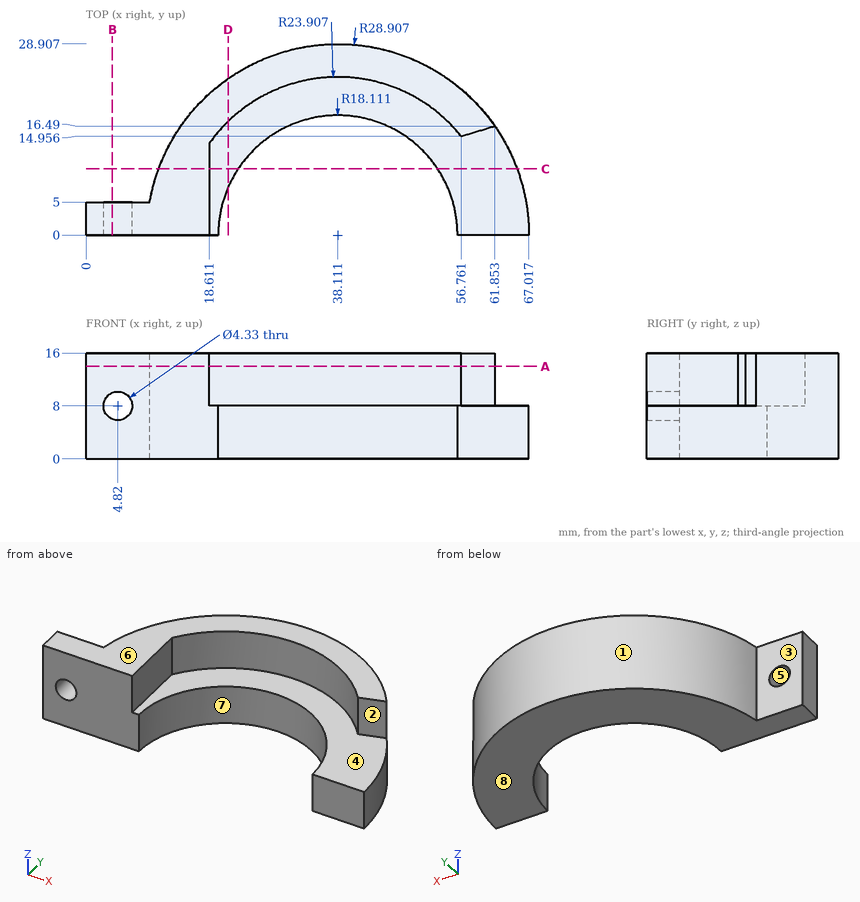
Geometry check sheet. Reference: drawing and pictorial views, mm from the part's lowest x, y, z. A direction names the side the tool comes from. Give positions to 0.01 mm unless a question says otherwise; leave off trailing zeros. Order: outer loops, then holes, each group sorted by start corner. A loop starts at its lowest first (then second) coordinate and runs counter-clockwise, first axis right, second up. Notation, with made-up numbers: M 17,45.25 L 68,45.25 A12 ccw 68,66.25 Z; hole C -20.5,9.5 d8. An arc over 180 degrees is marked long. Return JSON: item names as keys, results as strings. Group by question number.
1) Access from +Z, -Z, +X, -X, +Y, -Y to the whole of each face (thin tool, end or side, straight path). Record for the marked faces 1, 2, 3 and 4.
2) Section check D-D on x = 21.5. Record the cut outline in (y, z), and give its area (3 significant figures).
3) Scan lines: line 1 (Z direction, x = 47, y = 16.25); line 2 (X direction, y = 11.75, z = 6.75); line 3 (Y direction, x = 9.5, z = 9). Record each from-to range of solid material in increasing order.
4) Section check B-B on x = 4. Record the cut outline in (y, z).
5) Mould release check, pull along Z, two halves, no side actions. Record for the marked faces 5, 6, 7 and 8: pulls with the +Z half, pulls with the -Z half, needs draft (parallel to the pull), parting line crosses it, or undercut.
6) Section check A-A on z = 14. Record the cut outline in (x, y) (1 decimal), and give its area (3 significant figures).
7) Go/stop test with flat-tipped pins: pin 1 Ø4 at (x, y) = (34, 16.5) entering from +Z; pin 2 Ø12 at (x, y) = (51.5, 12.5) entering from +Z; pin 3 Ø2 at (y, z) = (17, 4.5) entering from -X (1 decimal); pin 4 Ø8 at (y, z) = (12.5, 6.5) entering from -X. Record where each tip stops, or that it passes through.
8) Section check C-C on y = 10. Record the cut outline in (x, z).
Answer block:
{
 "1": {"face 1": "+Z, -Z, +Y", "face 2": "+Z, +X, -Y", "face 3": "+Z, -Z, -X, +Y", "face 4": "+Z, -Y"},
 "2": {"outline": "M 7.22,0 L 23.66,0 L 23.66,16 L 17.19,16 L 17.19,8 L 7.22,8 Z", "area": "183 mm^2"},
 "3": {"line 1": "z = 0 to 8", "line 2": "x = 11.7 to 24.33, 51.89 to 64.52", "line 3": "y = 0 to 5"},
 "4": {"outline": "M 0,0 L 5,0 L 5,6 L 0,6 Z; M 0,10 L 5,10 L 5,16 L 0,16 Z"},
 "5": {"face 5": "undercut", "face 6": "pulls with the +Z half", "face 7": "needs draft", "face 8": "pulls with the -Z half"},
 "6": {"outline": "M 0,0 L 18.6,0 L 18.6,13.8 A23.9 cw 56.8,15 L 61.9,16.5 A28.9 ccw 9.6,5 L 0,5 Z", "area": "419 mm^2"},
 "7": {"pin 1": "stops at z = 8", "pin 2": "stops at z = 16", "pin 3": "stops at x = 14", "pin 4": "stops at x = 10.48"},
 "8": {"outline": "M 10.99,0 L 23.01,0 L 23.01,8 L 18.61,8 L 18.61,16 L 10.99,16 Z; M 53.21,0 L 65.23,0 L 65.23,8 L 53.21,8 Z"}
}
